For this review, take the finished solid that the model builds, in its own axes (mm). A direction names the side the tool comes from. Give positions to 0.01 mm unless a question says otherwise; leave off trailing zeros. Loops run counter-clockwise (first coordinate to the right, second up) from the corner with the lowest first, then second, coordinate; pieces in that order, holes last. Notation, with made-up numbers: (-1.5, 41.5) - (26.5, 41.5) arc R4 ccw to (26.5, 46.5) - close; hole circle Ø7 at (54.5, -10). An arc over 180 degrees is marked (long way). Use CSV: the item, a comma, the result in double quotes. Start each with the question number.
1. For pin 1 (5 mm diameter, centred on x = -182.5, z = 468, fed in from -Y); pin 2 (7.5 mm diameter, centred on x = 99.5, y = -183.5, fed in from +Z); pin 3 (7.5 mm diameter, centred on y = -184.5, z = 675, fed in from -X), all flat-tipped, find the tip position at first contact; note any pin that passes through.
2. Mouldability with a two-part tool opening along X and no side actions: class faces 5 (the flat face through (-298, -160, 355)), 6 (the flat face through (252, -182, 88.5)), 7 (the flat face through (-4, -2, 698)) as pulls with the +X half, pulls with the -X half, needs draft (parallel to the pull), parting line crosses it, or undercut.
3. Take a section at C-C on z = 614.5. Give the boundary of the cut face in (x, y).
4. Take a section at D-D on x = 101. Give the boundary of the cut face in (y, z), plus the area to 3 significant figures.
5. Take a section at B-B on x = -243. Give the boundary of the cut face in (y, z).
6. Wall thickness on line 1 (Z direction, x = 128, y = 27.5); line 2 (X direction, y = 68.5, z = 176); line 3 (Z direction, x = 154, y = -172.5): over which ranges is each line inside the solid? List them lowest first.
7. For faces 1 (the flat face through (278, -2, 355)), 2 (the flat face through (-4, -182, 713)), 3 (the flat face through (-4, -182, 87)), 4 (the flat face through (-293, -182, 672)), list the 3-axis set-ups (+Z, -Z, +X, -X, +Y, -Y) from which the entire face can be reached by the end or side of a thin tool; tool diameter is ignored.
8. Take a section at A-A on y = 58.5. Give the boundary of the cut face in (x, z).
```python
from build123d import *

# Parameters (mm, degrees)
F0_W     = 600
F0_H     = 300
F1_DEPTH = 720
F2_W     = 556
F2_H     = 676
F3_DEPTH = 300
F4_W     = 596
F4_H     = 716
F5_DEPTH = 20
F6_W     = 586
F6_H     = 80
F6_W_2   = 80
F6_H_2   = 543
F7_DEPTH = 25


with BuildPart() as f1:
    # F0 (on Top) → F1 (new body)
    with BuildSketch(Plane.XY):
        Rectangle(F0_W, F0_H)
    extrude(amount=F1_DEPTH)

    # F2 (on face) → F3 (cut, through all)
    with BuildSketch(Plane.XZ.offset(150)):
        with Locations((0, 360)):
            Rectangle(F2_W, F2_H)
    extrude(amount=-F3_DEPTH, mode=Mode.SUBTRACT)

    # F4 (on face) → F5 (join)
    with BuildSketch(Plane.XZ.offset(150)):
        with Locations((0, 360)):
            Rectangle(F4_W, F4_H)
    extrude(amount=F5_DEPTH)

    # F6 (on face) → F7 (join)
    with BuildSketch(Plane.XZ.offset(170)):
        with Locations((0, 673)):
            Rectangle(F6_W, F6_H)
        with Locations((-253, 360)):
            Rectangle(F6_W_2, F6_H_2)
        with Locations((253, 360)):
            Rectangle(F6_W_2, F6_H_2)
        with Locations((0, 47)):
            Rectangle(F6_W, F6_H)
    extrude(amount=F7_DEPTH)


solid = f1.part
```
Check result:
1,pin 1,"stops at y = -170"
1,pin 2,"stops at z = 713"
1,pin 3,"stops at x = -293"
2,face 5,"pulls with the -X half"
2,face 6,"needs draft"
2,face 7,"undercut"
3,outline,"(-300, -150) - (-298, -150) - (-298, -170) - (-293, -170) - (-293, -195) - (-213, -195) - (-213, -170) - (213, -170) - (213, -195) - (293, -195) - (293, -170) - (298, -170) - (298, -150) - (300, -150) - (300, 150) - (278, 150) - (278, -150) - (-278, -150) - (-278, 150) - (-300, 150) - close"
4,outline,"(-195, 7) - (-170, 7) - (-170, 2) - (-150, 2) - (-150, 0) - (150, 0) - (150, 22) - (-150, 22) - (-150, 698) - (150, 698) - (150, 720) - (-150, 720) - (-150, 718) - (-170, 718) - (-170, 713) - (-195, 713) - (-195, 633) - (-170, 633) - (-170, 87) - (-195, 87) - close"
4,area,"31,500 mm²"
5,outline,"(-195, 7) - (-170, 7) - (-170, 2) - (-150, 2) - (-150, 0) - (150, 0) - (150, 22) - (-150, 22) - (-150, 698) - (150, 698) - (150, 720) - (-150, 720) - (-150, 718) - (-170, 718) - (-170, 713) - (-195, 713) - (-195, 633) - (-170, 633) - (-170, 631.5) - (-195, 631.5) - (-195, 88.5) - (-170, 88.5) - (-170, 87) - (-195, 87) - close"
6,line 1,"z = 0 to 22, 698 to 720"
6,line 2,"x = -300 to -278, 278 to 300"
6,line 3,"z = 7 to 87, 633 to 713"
7,face 1,"+Y"
7,face 2,"+Z, +X, -X, -Y"
7,face 3,"+X, -X, -Y"
7,face 4,"+Z, -Z, -X, -Y"
8,outline,"(-300, 0) - (300, 0) - (300, 720) - (-300, 720) - close; hole (-278, 22) - (278, 22) - (278, 698) - (-278, 698) - close"
